Part model, mm, in its own coordinate system. A direction names the side the tool comes from. Round coordinates to 2 decimals unless told otherwise and drop trailing zeros. Loops run counter-clockwise (first coordinate to the right, second up) from the corner with the lowest first, then second, coordinate; pieces in that order, holes last. Notation, with made-up numbers: M 17.5,10.5 L 54.5,10.5 A17 ccw 54.5,30.5 Z; hole C 75,-9.75 d11. An arc over 180 degrees is marked long. Write each question's results on one line, items separated by ' | '.
from build123d import *

# Parameters (mm, degrees)
F0_W          = 151.9167423248
F0_H          = 152.3730680346
F1_DEPTH      = 101.6
F1_DEPTH_BACK = 101.6
F3_D          = 151.892
F3_DEPTH      = 203.2
F3_TIP        = 45.6329605727
F4_W          = 153.0907899141
F4_H          = 202.4234843612
F5_DEPTH      = 0.254


with BuildPart() as f1:
    # F0 (on Top) → F1 (new body, two sides)
    with BuildSketch(Plane.XY) as f1_sk:
        with Locations((-0.2950653434, 0.2231635153)):
            Rectangle(F0_W, F0_H)
    extrude(amount=F1_DEPTH)
    extrude(f1_sk.sketch, amount=-F1_DEPTH_BACK)

    # F3
    with Locations(Plane.XY.offset(101.6)):
        with Locations((0, 0)):
            Hole(F3_D / 2, depth=F3_DEPTH)
            with Locations((0, 0, -(F3_DEPTH + F3_TIP / 2))):  # 118° drill point
                Cone(0, F3_D / 2, F3_TIP, mode=Mode.SUBTRACT)

    # F4 (on face) → F5 (join)
    with BuildSketch(Plane.YZ.offset(75.663305819)):
        with Locations((0.5820244551, 0.3882578194)):
            Rectangle(F4_W, F4_H)
    extrude(amount=F5_DEPTH)


solid = f1.part
Item 1: Wall check: L1, parallel to X at y = 0, z = 58.5; L2, parallel to X at y = 44, z = -3.5; L3, parallel to Y at x = 12.5, z = -60. Give the ranges that are in metal, low to high.
Filled sheet:
L1: -76.25 to -75.95, 75.66 to 75.92 | L2: -76.25 to -61.9, 61.9 to 75.92 | L3: -75.96 to -74.91, 74.91 to 76.41
Item 2: Band-saw the part on A-A on y = 0. Give the cut face in (x, z), and give its area (3 significant figures).
Filled sheet:
outline: M -76.25,-101.6 L -75.95,-101.6 L -75.95,101.6 L -76.25,101.6 Z; M 75.66,-100.82 L 75.92,-100.82 L 75.92,101.6 L 75.66,101.6 Z | area: 114 mm^2
Item 3: Band-saw the part on C-C on z = -80. Give the cut face in (x, y), and give its area (3 significant figures).
Filled sheet:
outline: M -76.25,-75.96 L 75.92,-75.96 L 75.92,77.13 L 75.66,77.13 L 75.66,76.41 L -76.25,76.41 Z; hole M 75.66,-6.55 L 75.66,6.55 A75.95 ccw long Z | area: 5,070 mm^2
Item 4: Which spindle directions (+Z, -Z, +X, -X, +Y, -Y) get a long thin tool onto all of the face, cutting with end or side? Do faces 5 (the flat face through (-1, 76.41, 1)), 6 (the flat face through (-18, 74, -101.6)). Say none if no direction does.
Filled sheet:
face 5: +Z, -Z, -X, +Y | face 6: -Z, +X, -X, +Y, -Y
Item 5: Drop flat-ended pins along their axis: P1, Ø12, axis at x = -34.5, z = 51, coming from the +Y side; P2, Ø0.6, axis at y = 77, z = 14, coming from the -X side. Give the stop position or say it passes through.
Filled sheet:
P1: y = 76.41 | P2: x = 75.66
Item 6: Band-saw the part on D-D on y = -25. Give the cut face in (x, z), and give its area (3 significant figures).
Filled sheet:
outline: M -76.25,-101.6 L -71.71,-101.6 L -71.71,101.6 L -76.25,101.6 Z; M 71.71,-101.6 L 75.66,-101.6 L 75.66,-100.82 L 75.92,-100.82 L 75.92,101.6 L 71.71,101.6 Z | area: 1,780 mm^2
Item 7: Two-plate mould, pull along X, no slides. Class faces 1 (the cylindrical face through (-75.877, -3.248, -1.422)), 2 (the flat face through (-18, -75.963, -1)), 3 (the flat face through (-76.253, -1, 1)), 4 (the flat face through (75.663, 0, 2)): +X half, -X half, draft (parallel to the pull), parting line (faces both ways), or undercut.
Filled sheet:
face 1: undercut | face 2: draft | face 3: -X half | face 4: undercut
